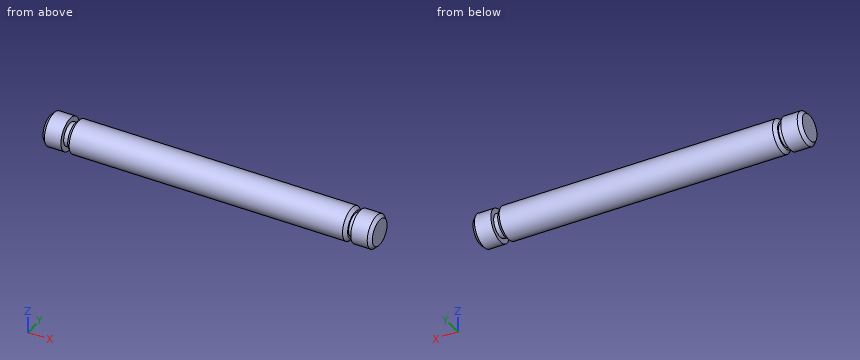
```python
from build123d import *

# Parameters (mm, degrees)
F2_SIZE = 1


with BuildPart() as f1:
    # F0 (on Front) → F1 (revolve)
    with BuildSketch(Plane.XZ):
        Polygon((-83.14801, 5), (-83.14801, 0), (16.85199, 0), (16.85199, 5), (10.85199, 5), (10.85199, 3.5), (9.35199, 3.5), (9.35199, 5), (-75.64801, 5), (-75.64801, 3.5), (-77.14801, 3.5), (-77.14801, 5), align=None)
    revolve(axis=Axis((-33.14801, 0, 0), (1, 0, 0)))

    # F2
    f2_edges = [f1.edges().sort_by_distance(p)[0] for p in [
        (-83.14801, 0, -5),
        (-75.64801, 0, -5),
        (16.85199, 0, -5),
        (9.35199, 0, -5),
    ]]
    chamfer(f2_edges, length=F2_SIZE)


solid = f1.part
```
Work out the finished part from the listing and answer in its coordinate system (mm). Coordinates: 2 decimals unless noted, no trailing zeros. Loops run counter-clockwise (first coordinate to the right, second up) from the corner with the lowest first, then second, coordinate; pieces in that order, holes last. Notation, with made-up numbers: M 7,-24 L 38,-24 A10 ccw 38,-17 Z; hole C 76,-2 d3. An arc over 180 degrees is marked long. Use CSV: the item, a comma, the result in double quotes. Start each with the question number.
(1) Consider line 1 (X direction, y = -2.5, z = 2.5); line 2 (X direction, y = -3.5, z = -3.25); line 3 (Y direction, x = -26, z = 3). Determine where each line is inside the solid, lowest interval first.
(2) Given pin 1 Ø1 at (y, z) = (-3, -3.5) entering from +X; pin 2 Ø3 at (x, y) = (-32, 2.5) entering from +Z; pin 3 Ø2 at (x, y) = (-53.5, -1.5) entering from +Z, each flat-ended and moving along its own axis, determine where each tip first touches the part or whether it passes through.
(3) Find section A-A, the plane x = -41.5. Give the vertices of the cut face in (y, z).
Recorded:
1,line 1,"x = -83.15 to -77.15, -75.65 to 9.35, 10.85 to 16.85"
1,line 2,"x = -82.37 to -77.15, -74.87 to 8.58, 10.85 to 16.08"
1,line 3,"y = -4 to 4"
2,pin 1,"stops at x = 16.74"
2,pin 2,"stops at z = 4.9"
2,pin 3,"stops at z = 4.97"
3,outline,"C 0,0 d10"
